from build123d import *

# Parameters (mm, degrees)
SKETCH2_R                                           = 25
SHELL2_T                                            = -3
SKETCH3_W                                           = 75
SKETCH3_H                                           = 75
SKETCH3_R                                           = 22
BOSS_EXTRUDE1_DEPTH                                 = 10
FILLET1_R                                           = 5
CBORE_FOR_8_BINDING_HEAD_MACHINE_SCREW1_D           = 4.4958
CBORE_FOR_8_BINDING_HEAD_MACHINE_SCREW1_DEPTH       = 20
CBORE_FOR_8_BINDING_HEAD_MACHINE_SCREW1_CBORE_D     = 9.525
CBORE_FOR_8_BINDING_HEAD_MACHINE_SCREW1_CBORE_DEPTH = 2.667
CBORE_FOR_8_BINDING_HEAD_MACHINE_SCREW1_TIP         = 1.350674586
SKETCH6_W                                           = 75
SKETCH6_H                                           = 75
SKETCH6_R                                           = 22
BOSS_EXTRUDE2_DEPTH                                 = 10
FILLET2_R                                           = 5
CBORE_FOR_8_BINDING_HEAD_MACHINE_SCREW2_D           = 4.4958
CBORE_FOR_8_BINDING_HEAD_MACHINE_SCREW2_DEPTH       = 20
CBORE_FOR_8_BINDING_HEAD_MACHINE_SCREW2_CBORE_D     = 9.525
CBORE_FOR_8_BINDING_HEAD_MACHINE_SCREW2_CBORE_DEPTH = 2.667
CBORE_FOR_8_BINDING_HEAD_MACHINE_SCREW2_TIP         = 1.350674586


with BuildPart() as part:
    # Sweep1: sweep along a path in Sketch1
    with BuildLine(Plane.XY) as sweep1_path:
        Line((-55, 50), (-55, 0))
        ThreePointArc((-55, 0), (-38.890872965, -38.890872965), (0, -55))
        Line((0, -55), (50, -55))
    # Sketch2 → Sweep1 (sweep)
    with BuildSketch(Plane(origin=(-55, 50, 0), x_dir=(-1, 0, 0), z_dir=(0, -1, 0))):
        with Locations((-0.233587872, 0)):
            Circle(SKETCH2_R)
    sweep(path=sweep1_path.line)

    # Shell2
    shell2_openings = [part.faces().sort_by_distance(p)[0] for p in [
        (50, -54.766412128, 0),
        (-54.766412128, 50, 0),
    ]]
    offset(amount=SHELL2_T, openings=shell2_openings, kind=Kind.INTERSECTION)

    # Sketch3 → Boss-Extrude1 (add)
    with BuildSketch(Plane(origin=(0, 50, 0), x_dir=(1, 0, 0), z_dir=(0, 1, 0))):
        with Locations((-54.766412128, 0)):
            Rectangle(SKETCH3_W, SKETCH3_H)
        with Locations(Location((-54.766412128, 0, 0), (0, 0, 180))):
            Circle(SKETCH3_R, mode=Mode.SUBTRACT)
    extrude(amount=BOSS_EXTRUDE1_DEPTH)

    # Fillet1
    fillet1_edges = [part.edges().sort_by_distance(p)[0] for p in [
        (-17.266412128, 55, 37.5),
        (-17.266412128, 55, -37.5),
        (-92.266412128, 55, -37.5),
        (-92.266412128, 55, 37.5),
    ]]
    fillet(fillet1_edges, radius=FILLET1_R)

    # CBORE for #8 Binding Head Machine Screw1
    with Locations(Plane(origin=(-80.88402288, 60, -26.197803089), x_dir=(0, 0, 1), z_dir=(0, 1, 0))):
        with Locations((0, 0), (0, 52.235221503), (52.395606178, 0), (52.395606178, 52.235221503)):
            CounterBoreHole(CBORE_FOR_8_BINDING_HEAD_MACHINE_SCREW1_D / 2, CBORE_FOR_8_BINDING_HEAD_MACHINE_SCREW1_CBORE_D / 2, CBORE_FOR_8_BINDING_HEAD_MACHINE_SCREW1_CBORE_DEPTH, depth=CBORE_FOR_8_BINDING_HEAD_MACHINE_SCREW1_DEPTH)
            with Locations((0, 0, -(CBORE_FOR_8_BINDING_HEAD_MACHINE_SCREW1_DEPTH + CBORE_FOR_8_BINDING_HEAD_MACHINE_SCREW1_TIP / 2))):  # 118° drill point
                Cone(0, CBORE_FOR_8_BINDING_HEAD_MACHINE_SCREW1_D / 2, CBORE_FOR_8_BINDING_HEAD_MACHINE_SCREW1_TIP, mode=Mode.SUBTRACT)

    # Sketch6 → Boss-Extrude2 (add)
    with BuildSketch(Plane(origin=(50, 0, 0), x_dir=(0, 0, -1), z_dir=(1, 0, 0))):
        with Locations((0, -54.766412128)):
            Rectangle(SKETCH6_W, SKETCH6_H)
        with Locations((0, -54.766412128)):
            Circle(SKETCH6_R, mode=Mode.SUBTRACT)
    extrude(amount=BOSS_EXTRUDE2_DEPTH)

    # Fillet2
    fillet2_edges = [part.edges().sort_by_distance(p)[0] for p in [
        (55, -92.266412128, -37.5),
        (55, -17.266412128, -37.5),
        (55, -17.266412128, 37.5),
        (55, -92.266412128, 37.5),
    ]]
    fillet(fillet2_edges, radius=FILLET2_R)

    # CBORE for #8 Binding Head Machine Screw2
    with Locations(Plane(origin=(60, 0, 0), x_dir=(0, 0, -1), z_dir=(1, 0, 0))):
        with Locations((-26.12, -80.966412128), (-26.12, -28.566412128), (26.12, -28.566412128), (26.12, -80.966412128)):
            CounterBoreHole(CBORE_FOR_8_BINDING_HEAD_MACHINE_SCREW2_D / 2, CBORE_FOR_8_BINDING_HEAD_MACHINE_SCREW2_CBORE_D / 2, CBORE_FOR_8_BINDING_HEAD_MACHINE_SCREW2_CBORE_DEPTH, depth=CBORE_FOR_8_BINDING_HEAD_MACHINE_SCREW2_DEPTH)
            with Locations((0, 0, -(CBORE_FOR_8_BINDING_HEAD_MACHINE_SCREW2_DEPTH + CBORE_FOR_8_BINDING_HEAD_MACHINE_SCREW2_TIP / 2))):  # 118° drill point
                Cone(0, CBORE_FOR_8_BINDING_HEAD_MACHINE_SCREW2_D / 2, CBORE_FOR_8_BINDING_HEAD_MACHINE_SCREW2_TIP, mode=Mode.SUBTRACT)


solid = part.part
Design review of the part built by this model. Coordinates are the model's own, in mm. A direction names the side the tool comes from. Coordinates: 2 decimals unless noted, no trailing zeros. Loops run counter-clockwise (first coordinate to the right, second up) from the corner with the lowest first, then second, coordinate; pieces in that order, holes last. Notation, with made-up numbers: (-16.75, 20.25) -> (-12.75, 20.25) arc R22 ccw to (-12.75, 59.25) -> close; hole circle Ø9 at (22.5, 33.25). An arc over 180 degrees is marked (long way). Use a Markdown table: item, result. Add a question column.
Item 1: Machinability: for faces 4 (the flat face through (-31, 57.333, 27)), 5 (the flat face through (-55, 55, -37.5)), 6 (the cylindrical face through (25.35, -78.61, -7.51)), 7 (the flat face through (-17.266, 55, 0)), 8 (the cylindrical face through (58.685, -85.616, -25.088)), which of the approach directions +Z, -Z, +X, -X, +Y, -Y give a long, thin tool a straight path to every point of the face, cutting with its end or side? Answer none if there is none.
Item 2: The part is to be moulded in two halves that separate along X. For faces 1 (the cylindrical face through (-28.55, 53.615, -23.952)), 2 (the cylindrical face through (53.615, -82.334, -27.904)), 3 (the cylindrical face through (-18.692, 55.07, -35.996)), say which applies: +X half, -X half, draft (parallel to the pull), parting line (faces both ways), or undercut.
Item 3: We need section B-B, the plane y = 26.5. Write out the cut boundary in (x, z).
Item 4: Wall thickness on L1, parallel to Y at x = 59, z = 26; L2, parallel to Y at x = 51, z = -26; L3, parallel to X at y = 47, z = 0: over which ranges is each line inside the solid? List them lowest first. Write a range as from..to.
Item 5: We need section A-A, the plane z = 0. Write out the cut boundary in (x, y), and give its area (3 significant figures).
Item 6: We need section C-C, the plane z = 9. Write out the cut boundary in (x, y), and give its area (3 significant figures).
Item 7: Clearance check with flat-ended pins moving along their axes: P1, Ø6, axis at y = 28.5, z = -17.5, coming from the +X side; P2, Ø8.5, axis at x = -80.88, z = -26.2, coming from the +Y side; P3, Ø8, axis at x = 31, z = 12.5, coming from the -Y side. State where each tip first meets the part, or that it passes through.
Numbers:
| question | item | result |
|---|---|---|
| 1 | face 4 | +Y |
| 1 | face 5 | -Z, +X, -X, +Y, -Y |
| 1 | face 6 | none |
| 1 | face 7 | +Z, -Z, +X, +Y |
| 1 | face 8 | +X |
| 2 | face 1 | undercut |
| 2 | face 2 | draft |
| 2 | face 3 | +X half |
| 3 | outline | circle Ø50 at (-54.77, 0); hole circle Ø44 at (-54.77, 0) |
| 4 | L1 | y = -92.27..-85.73, -76.21..-33.33, -23.81..-17.27 |
| 4 | L2 | y = -92.27..-83.21, -78.72..-30.81, -26.32..-17.27 |
| 4 | L3 | x = -79.77..-76.77, -32.77..-29.77 |
| 5 | outline | (-92.27, 50) -> (-79.77, 50) -> (-79.77, 0) arc R79.77 ccw to (0, -79.77) -> (50, -79.77) -> (50, -92.27) -> (60, -92.27) -> (60, -76.77) -> (0, -76.77) arc R76.77 cw to (-76.77, 0) -> (-76.77, 60) -> (-92.27, 60) -> close; (-32.77, 0) arc R32.77 ccw to (0, -32.77) -> (60, -32.77) -> (60, -17.27) -> (50, -17.27) -> (50, -29.77) -> (0, -29.77) arc R29.77 cw to (-29.77, 0) -> (-29.77, 50) -> (-17.27, 50) -> (-17.27, 60) -> (-32.77, 60) -> close |
| 5 | area | 1,740 mm^2 |
| 6 | outline | (-92.27, 50) -> (-78.09, 50) -> (-78.09, 0) arc R78.09 ccw to (0, -78.09) -> (50, -78.09) -> (50, -92.27) -> (60, -92.27) -> (60, -74.84) -> (0, -74.84) arc R74.84 cw to (-74.84, 0) -> (-74.84, 60) -> (-92.27, 60) -> close; (-34.69, 0) arc R34.69 ccw to (0, -34.69) -> (60, -34.69) -> (60, -17.27) -> (50, -17.27) -> (50, -31.44) -> (0, -31.44) arc R31.44 cw to (-31.44, 0) -> (-31.44, 50) -> (-17.27, 50) -> (-17.27, 60) -> (-34.69, 60) -> close |
| 6 | area | 1,910 mm^2 |
| 7 | P1 | stops at x = -34.4 |
| 7 | P2 | stops at y = 57.33 |
| 7 | P3 | stops at y = -78.28 |
